Check sheet for the modelled part. Datum: model origin and axes. Units: mm. A direction names the side the tool comes from. Round coordinates to 2 decimals unless told otherwise and drop trailing zeros. Write each loop counter-clockwise with the first axis right and the second up, starting at its lowest first coordinate (ties: lowest second). Pieces come first, ordered by that corner, then holes. Notation, with made-up numbers: (54.5, 76) - (102.5, 76) arc R28 ccw to (102.5, 94) - close; hole circle Ø8 at (-26, -22.5). An arc over 180 degrees is marked (long way). Answer as a JSON object with one key per item and string values. Group by question number.
Item 1: Sectioned sample at B-B on z = 10.75. Record the boundary of the cut face in (x, y).
Item 2: Sectioned sample at A-A on y = 19.05. Record the boundary of the cut face in (x, z).
Item 3: Sectioned sample at C-C on z = 18. Record the boundary of the cut face in (x, y).
Item 4: Thickness scan on line 1 (X direction, y = 4.5, z = 7.75); line 2 (Z direction, x = 11.5, y = -5); line 3 (Z direction, x = 22, y = -20). Record the ranges inside material, lowest first.
Item 5: Gauge pin test, flat ends, axial feed: P1, Ø8.5, axis at x = 1, z = 2.5, coming from the +Y side; P2, Ø1.2, axis at x = -23.5, y = 15.5, coming from the -Z side; P3, Ø8, axis at x = -3.5, y = 4.5, coming from the +Z side. Record the tip position at first contact, or that the pin passes through.
Item 6: Set-up check for faces 5 (the flat face through (0, 6.35, -1)), 6 (the flat face through (-24, 31.75, 18)), 7 (the flat face through (-22.987, -7, 14)): record each of +Z, -Z, +X, -X, +Y, -Y from which the full face is reachable in a straight line by a thin tool's end or side.
Item 7: Release check for a two-part mould opening along X. For faces 1 (the flat face through (-24.511, -7, 13)), 2 (the flat face through (24, 19, 9.398)), 3 (the flat face through (22.987, -8, 14)), 4 (the cylindrical face through (23.594, -12.967, -0.655)) record: pulls with the +X half, pulls with the -X half, needs draft (parallel to the pull), parting line crosses it, or undercut.
Item 8: Sectioned sample at D-D on y = 26. Record the boundary of the cut face in (x, z), plus the area to 3 significant figures.
```python
from build123d import *

# Parameters (mm, degrees)
CROQUIS1_W                         = 49.022
CROQUIS1_H                         = 63.5
BRIDA_BASE1_DEPTH                  = 1.524
BRIDA_DE_ARISTA1_STRIP_W           = 9.144
BRIDA_DE_ARISTA1_STRIP_H           = 1.524
BRIDA_DE_ARISTA1_STRIP_CUT_DEPTH   = 63.5
BRIDA_DE_ARISTA1_STRIP_2_W         = 9.144
BRIDA_DE_ARISTA1_STRIP_2_H         = 1.524
BRIDA_DE_ARISTA1_STRIP_CUT_2_DEPTH = 63.5
BRIDA_DE_ARISTA1_DEPTH             = 63.5
BRIDA_DE_ARISTA1_BEND_DEPTH        = 63.5
CROQUIS23_R                        = 3.175
CROQUIS23_W                        = 10.922
CROQUIS23_H                        = 25.4
CORTAR_EXTRUIR4_DEPTH              = 73.66


# Sheet-metal steps are written as plain solids
with BuildPart() as part:
    # Croquis1 → Brida base1 (new body)
    with BuildSketch(Plane.XY):
        Rectangle(CROQUIS1_W, CROQUIS1_H)
    extrude(amount=-BRIDA_BASE1_DEPTH)

    # Brida de arista1 strip (across the edge) → Brida de arista1 strip cut (cut)
    with BuildSketch(Plane(origin=(24.511, -31.75, 0), x_dir=(-1, 0, 0), z_dir=(0, 1, 0))):
        with Locations((-1.524, -0.762)):
            Rectangle(BRIDA_DE_ARISTA1_STRIP_W, BRIDA_DE_ARISTA1_STRIP_H)
    extrude(amount=BRIDA_DE_ARISTA1_STRIP_CUT_DEPTH, mode=Mode.SUBTRACT)

    # Brida de arista1 strip 2 (across the edge) → Brida de arista1 strip cut 2 (cut)
    with BuildSketch(Plane(origin=(-24.511, 31.75, 0), x_dir=(1, 0, 0), z_dir=(0, -1, 0))):
        with Locations((-1.524, -0.762)):
            Rectangle(BRIDA_DE_ARISTA1_STRIP_2_W, BRIDA_DE_ARISTA1_STRIP_2_H)
    extrude(amount=BRIDA_DE_ARISTA1_STRIP_CUT_2_DEPTH, mode=Mode.SUBTRACT)

    # Brida de arista1 section (across the edge) → Brida de arista1 (add)
    with BuildSketch(Plane(origin=(24.511, -31.75, 0), x_dir=(-1, 0, 0), z_dir=(0, 1, 0))):
        with BuildLine():
            Line((0, 1.524), (0, 25.4))
            Line((0, 25.4), (1.524, 25.4))
            Line((1.524, 25.4), (1.524, 1.524))
            ThreePointArc((1.524, 1.524), (1.970369265, 0.446369265), (3.048, 0))
            Line((3.048, 0), (3.048, -1.524))
            ThreePointArc((3.048, -1.524), (0.892738531, -0.631261469), (0, 1.524))
        make_face()
    extrude(amount=BRIDA_DE_ARISTA1_DEPTH)

    # Brida de arista1 section 2 (across the edge) → Brida de arista1 bend (add)
    with BuildSketch(Plane(origin=(-24.511, 31.75, 0), x_dir=(1, 0, 0), z_dir=(0, -1, 0))):
        with BuildLine():
            Line((0, 1.524), (0, 25.4))
            Line((0, 25.4), (1.524, 25.4))
            Line((1.524, 25.4), (1.524, 1.524))
            ThreePointArc((1.524, 1.524), (1.970369265, 0.446369265), (3.048, 0))
            Line((3.048, 0), (3.048, -1.524))
            ThreePointArc((3.048, -1.524), (0.892738531, -0.631261469), (0, 1.524))
        make_face()
    extrude(amount=BRIDA_DE_ARISTA1_BEND_DEPTH)

    # Croquis23 → Cortar-Extruir4 (cut)
    with BuildSketch(Plane(origin=(24.511, 0, 0), x_dir=(0, 0, -1), z_dir=(1, 0, 0))):
        with Locations((-17.4752, 19.05)):
            Circle(CROQUIS23_R)
        with Locations((-3.937, 19.05)):
            Rectangle(CROQUIS23_W, CROQUIS23_H)
    extrude(amount=-CORTAR_EXTRUIR4_DEPTH, mode=Mode.SUBTRACT)


solid = part.part
```
Completed:
{
 "1": {"outline": "(-24.51, -31.75) - (-22.99, -31.75) - (-22.99, 31.75) - (-24.51, 31.75) - close; (22.99, -31.75) - (24.51, -31.75) - (24.51, 31.75) - (22.99, 31.75) - close"},
 "2": {"outline": "(-24.51, 9.4) - (-22.99, 9.4) - (-22.99, 14.3) - (-24.51, 14.3) - close; (-24.51, 20.65) - (-22.99, 20.65) - (-22.99, 25.4) - (-24.51, 25.4) - close; (22.99, 9.4) - (24.51, 9.4) - (24.51, 14.3) - (22.99, 14.3) - close; (22.99, 20.65) - (24.51, 20.65) - (24.51, 25.4) - (22.99, 25.4) - close"},
 "3": {"outline": "(-24.51, -31.75) - (-22.99, -31.75) - (-22.99, 15.92) - (-24.51, 15.92) - close; (-24.51, 22.18) - (-22.99, 22.18) - (-22.99, 31.75) - (-24.51, 31.75) - close; (22.99, -31.75) - (24.51, -31.75) - (24.51, 15.92) - (22.99, 15.92) - close; (22.99, 22.18) - (24.51, 22.18) - (24.51, 31.75) - (22.99, 31.75) - close"},
 "4": {"line 1": "-24.51 to -22.99, 22.99 to 24.51", "line 2": "-1.52 to 0", "line 3": "-1.48 to 0.1"},
 "5": {"P1": "y = 6.35", "P2": "z = 9.4", "P3": "z = 0"},
 "6": {"face 5": "-Z, +X, -X, +Y", "face 6": "+Z, -Z, +X, -X, +Y", "face 7": "+Z, +Y, -Y"},
 "7": {"face 1": "pulls with the -X half", "face 2": "needs draft", "face 3": "undercut", "face 4": "pulls with the +X half"},
 "8": {"outline": "(-24.51, 9.4) - (-22.99, 9.4) - (-22.99, 25.4) - (-24.51, 25.4) - close; (22.99, 9.4) - (24.51, 9.4) - (24.51, 25.4) - (22.99, 25.4) - close", "area": "48.8 mm²"}
}
